Verification items for the finished model (mm, model axes). A direction names the side the tool comes from. Give positions to 0.01 mm unless a question says otherwise; leave off trailing zeros. Loops run counter-clockwise (first coordinate to the right, second up) from the corner with the lowest first, then second, coordinate; pieces in that order, holes last. Notation, with made-up numbers: (-10, -20) -> (12, -20) arc R19 cw to (12, -1) -> close; hole circle Ø10 at (10, 67). An arc over 180 degrees is marked (long way). Use one line per item in the form item = value. Start each with the question number.
from build123d import *

# Parameters (mm, degrees)
SKETCH1_R           = 7.4
LENS_BODY_DEPTH     = 8
SKETCH2_R           = 7.4
LENS_SHOULDER_DEPTH = 3
LENS_SHOULDER_TAPER = 30
SKETCH3_R           = 5.667949192
LENS_CROWN_DEPTH    = 3.2
LENS_CROWN_TAPER    = 50
SKETCH4_R           = 2.6
LED_CAVITY_DEPTH    = 4.75


with BuildPart() as part:
    # Sketch1 → Lens_body (new body)
    with BuildSketch(Plane.XY):
        Circle(SKETCH1_R)
    extrude(amount=LENS_BODY_DEPTH)

    # Sketch2 → Lens_shoulder (add)
    with BuildSketch(Plane.XY.offset(8)):
        Circle(SKETCH2_R)
    extrude(amount=LENS_SHOULDER_DEPTH, taper=LENS_SHOULDER_TAPER)

    # Sketch3 → Lens_crown (add)
    with BuildSketch(Plane.XY.offset(11)):
        Circle(SKETCH3_R)
    extrude(amount=LENS_CROWN_DEPTH, taper=LENS_CROWN_TAPER)

    # Sketch4 → LED_cavity (cut, symmetric)
    with BuildSketch(Plane.XY.offset(4.25)):
        Circle(SKETCH4_R)
    extrude(amount=LED_CAVITY_DEPTH, both=True, mode=Mode.SUBTRACT)


solid = part.part
Item 1: Tool access check on faces 4 (the flat face through (0, 0, 9)), 5 (the conical face through (-1.618, -1.241, 14.045)). Record the directions out of +Z, -Z, +X, -X, +Y, -Y that give a thin tool (end or side, any length) a straight path to the whole face; none if there is none.
Item 2: Material ranges on line 1 (Y direction, x = 0, z = 5); line 2 (X direction, y = -2, z = 13); line 3 (Y direction, x = 1.75, z = 7), recorded low to high.
Item 3: Gauge pin test, flat ends, axial feed: pin 1 Ø3 at (x, y) = (0, 0) entering from -Z; pin 2 Ø1.5 at (x, y) = (-4.5, -4.5) entering from +Z; pin 3 Ø6 at (x, z) = (-5, 5) entering from -Y. Record the tip position at first contact, or that the pin passes through.
Item 4: Sectioned sample at C-C, the plane z = 10.75. Enter the section's corners in (x, y), and give its area (3 significant figures).
Item 5: Sectioned sample at A-A, the plane y = 0. Enter the section's corners in (x, z).
Item 6: Draft check along X on faces 1 (the cylindrical face through (-1.604, -7.224, 3.944)), 2 (the flat face through (0, 0, 14.2)), 3 (the cylindrical face through (-0.338, 2.578, 4.563)). Enter one of: +X half, -X half, draft (parallel to the pull), parting line (faces both ways), or undercut.
Outcome:
q1.face_4 = -Z
q1.face_5 = +Z
q2.line_1 = -7.4 to -2.6, 2.6 to 7.4
q2.line_2 = -2.61 to 2.61
q2.line_3 = -7.19 to -1.92, 1.92 to 7.19
q3.pin_1 = 9
q3.pin_2 = 11.05
q3.pin_3 = -7.12
q4.outline = circle Ø11.62 at (0, 0)
q4.area = 106 mm^2
q5.outline = (-7.4, 0) -> (-2.6, 0) -> (-2.6, 9) -> (2.6, 9) -> (2.6, 0) -> (7.4, 0) -> (7.4, 8) -> (5.67, 11) -> (1.85, 14.2) -> (-1.85, 14.2) -> (-5.67, 11) -> (-7.4, 8) -> close
q6.face_1 = parting line
q6.face_2 = draft
q6.face_3 = undercut
